Could you check a few things on this drawing? It's one solid part, dimensions in mm from its lowest x, y, z. Round coordinates to 2 decimals unless told otherwise and drop trailing zeros. Loops run counter-clockwise (first coordinate to the right, second up) from the corner with the lowest first, then second, coordinate; pieces in that order, holes last. Notation, with made-up numbers: M 78.25,56 L 103.25,56 A29 ccw 103.25,86 Z; hole C 79.25,48 d11. An arc over 180 degrees is marked long. Write item = value, one per line. Start each with the question number.
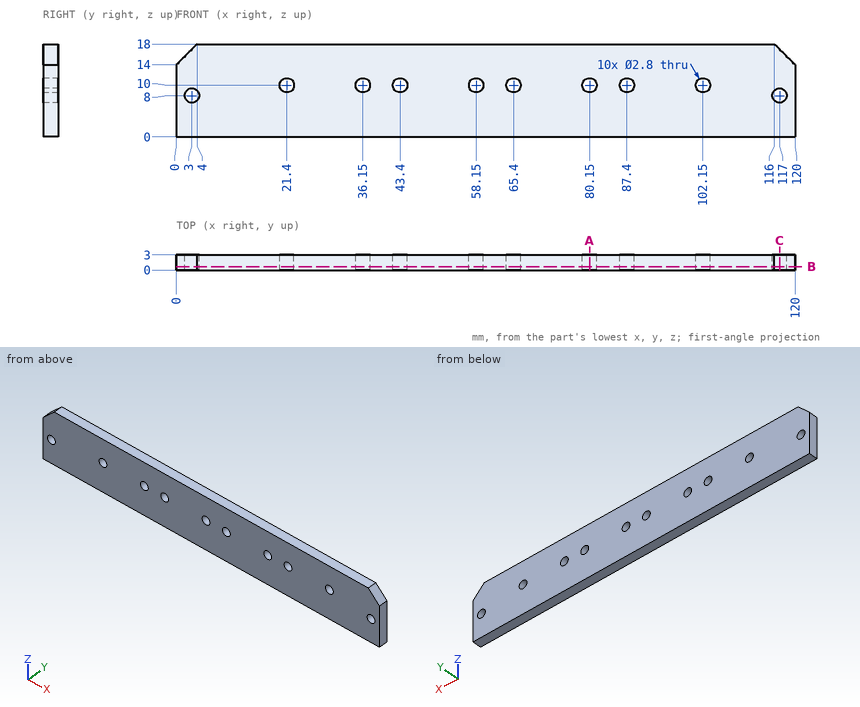
Item 1: I want a section at B-B, the plane y = 0.7. State how many separate pieces and enclosed holes the cut face has, then the cut area to 3 significant figures.
Item 2: I want a section at A-A, the plane x = 80.15. List the corners of the cut face in (y, z) for me.
Item 3: I want a section at C-C, the plane x = 117. List the corners of the cut face in (y, z) for me, then the cut area to 3 significant figures.
Item 4: Please list where these lines run through material, in increasing order: line 1 (X direction, y = 2.15, z = 7.75); line 2 (X direction, y = 1.3, z = 7.5); line 3 (Z direction, x = 117, y = 1.7). Write a range as [from, to].
Worked out:
q1.separate_pieces = 1
q1.enclosed_holes = 10
q1.area = 2,080 mm2
q2.outline = M 0,0 L 3,0 L 3,8.6 L 0,8.6 Z; M 0,11.4 L 3,11.4 L 3,18 L 0,18 Z
q3.outline = M 0,0 L 3,0 L 3,6.6 L 0,6.6 Z; M 0,9.4 L 3,9.4 L 3,17 L 0,17 Z
q3.area = 42.6 mm2
q4.line_1 = [0, 1.62], [4.38, 115.62], [118.38, 120]
q4.line_2 = [0, 1.69], [4.31, 115.69], [118.31, 120]
q4.line_3 = [0, 6.6], [9.4, 17]
